Source: CAD feature listing. Evaluate the final solid. Frame: model axes, mm. A direction names the side the tool comes from. Give positions to 0.01 mm unless a question says otherwise; leave off trailing zeros. Loops run counter-clockwise (first coordinate to the right, second up) from the corner with the lowest first, then second, coordinate; pieces in that order, holes last. Notation, with made-up numbers: M -16,-31.75 L -10,-31.75 A24 cw -10,1.25 Z; hole C 36,53 d8. An arc over 180 degrees is marked long. Answer in a Markdown table with one row per item.
```python
from build123d import *

# Parameters (mm, degrees)
F1_DEPTH = 19.05
F2_R     = 1.5875
F3_DEPTH = 1.651


with BuildPart() as f1:
    # F0 (on Front) → F1 (new body)
    with BuildSketch(Plane.XZ):
        with BuildLine():
            Line((0, 6.35), (0, 0))
            ThreePointArc((0, 0), (-0.36356, -0.690866), (-1.138859, -0.782422))
            Line((-1.138859, -0.782422), (-3.175, 0))
            Line((-3.175, 0), (-11.811, 0))
            ThreePointArc((-11.811, 0), (-12.439618, -0.260382), (-12.7, -0.889))
            Line((-12.7, -0.889), (-12.7, -2.286))
            ThreePointArc((-12.7, -2.286), (-12.439618, -2.914618), (-11.811, -3.175))
            Line((-11.811, -3.175), (-0.8382, -3.175))
            ThreePointArc((-0.8382, -3.175), (1.406864, -2.245064), (2.3368, 0))
            Line((2.3368, 0), (2.3368, 6.35))
            ThreePointArc((2.3368, 6.35), (1.406864, 8.595064), (-0.8382, 9.525))
            Line((-0.8382, 9.525), (-11.811, 9.525))
            ThreePointArc((-11.811, 9.525), (-12.439618, 9.264618), (-12.7, 8.636))
            Line((-12.7, 8.636), (-12.7, 7.239))
            ThreePointArc((-12.7, 7.239), (-12.439618, 6.610382), (-11.811, 6.35))
            Line((-11.811, 6.35), (-3.175, 6.35))
            Line((-3.175, 6.35), (-1.138859, 7.132422))
            ThreePointArc((-1.138859, 7.132422), (-0.36356, 7.040866), (0, 6.35))
        make_face()
    extrude(amount=F1_DEPTH)

    # F2 (on face) → F3 (cut)
    with BuildSketch(Plane(origin=(0, 0, -3.175), x_dir=(1, 0, 0), z_dir=(0, 0, -1))):
        with Locations((-6.35, 15.875)):
            Circle(F2_R)
        with Locations((-6.35, 3.175)):
            Circle(F2_R)
        with Locations((-6.35, 9.525)):
            Circle(F2_R)
    extrude(amount=-F3_DEPTH, mode=Mode.SUBTRACT)


solid = f1.part
```
1) Pull-direction query (X, two-part tool) for faces 1 (the flat face through (-6, -3, -1.524)), 2 (the cylindrical face through (-12.4, -9.4, 9.3)), 3 (the flat face through (-7, -9, 0)), 4 (the flat face through (-2.143, -9.392, -0.397)); classes: released by +X, released by -X, zero draft, split by the parting line, or undercut.
Reply:
| item | result |
|---|---|
| face 1 | undercut |
| face 2 | released by -X |
| face 3 | zero draft |
| face 4 | undercut |
2) Section B-B, the plane y = -16.5. Return loops of the section in (x, z) (3 decimals), then the cut area to 3 significant figures.
Reply:
| item | result |
|---|---|
| outline | M -12.7,-2.286 A0.889 ccw -11.811,-3.175 L -7.809,-3.175 L -7.809,-1.524 L -4.891,-1.524 L -4.891,-3.175 L -0.838,-3.175 A3.175 ccw 2.337,0 L 2.337,6.35 A3.175 ccw -0.838,9.525 L -11.811,9.525 A0.889 ccw -12.7,8.636 L -12.7,7.239 A0.889 ccw -11.811,6.35 L -3.175,6.35 L -1.139,7.132 A0.838 cw 0,6.35 L 0,0 A0.838 cw -1.139,-0.782 L -3.175,0 L -11.811,0 A0.889 ccw -12.7,-0.889 Z |
| area | 97.3 mm² |
3) Set-up query: faces 5 (the cylindrical face through (-12.43, -9.39, -0.25)), 6 (the cylindrical face through (-0.35, -9.39, -0.68)), 7 (the cylindrical face through (-12.446, -9.392, -2.908)), 8 (the flat face through (-6, -10, -1.524)), 9 (the flat face through (2.337, -9, 3)). Return all of +Z, -Z, +X, -X, +Y, -Y with unobstructed straight access to the full face (end or side cutting, diameter ignored); none if empty.
Reply:
| item | result |
|---|---|
| face 5 | -X, +Y, -Y |
| face 6 | +Y, -Y |
| face 7 | -Z, -X, +Y, -Y |
| face 8 | -Z |
| face 9 | +Z, -Z, +X, +Y, -Y |
4) Pin query (flat end, axial travel): pin 1 Ø1.6 at (x, y) = (-6, -16.5) entering from -Z; pin 2 Ø3 at (y, z) = (-10, 4) entering from -X. Return the tip coordinate at first contact, or that it passes through.
Reply:
| item | result |
|---|---|
| pin 1 | stops at z = -1.52 |
| pin 2 | stops at x = 0 |
5) Section D-D, the plane x = -2.75. Return loops of the section in (y, z) (3 decimals).
Reply:
| item | result |
|---|---|
| outline | M -19.05,-3.175 L 0,-3.175 L 0,-0.163 L -19.05,-0.163 Z; M -19.05,6.513 L 0,6.513 L 0,9.525 L -19.05,9.525 Z |
6) Section C-C, the plane z = 3.25. Return loops of the section in (x, y), then the cut area to 3 significant figures.
Reply:
| item | result |
|---|---|
| outline | M 0,-19.05 L 2.34,-19.05 L 2.34,0 L 0,0 Z |
| area | 44.5 mm² |
7) Material intervals for L1, parallel to Y at x = -6.35, z = -2.75; L2, parallel to Z at x = -9.5, y = -9 (3 decimals); L3, parallel to Z at x = -7.5, y = -8.75 (3 decimals), sorted ascending.
Reply:
| item | result |
|---|---|
| L1 | y = -19.05 to -17.46, -14.29 to -11.11, -7.94 to -4.76, -1.59 to 0 |
| L2 | z = -3.175 to 0, 6.35 to 9.525 |
| L3 | z = -1.524 to 0, 6.35 to 9.525 |
